Geometry: see drawing. Coordinates: mm, zero at the bounding-box minimum. A direction names the side the tool comes from. Round coordinates to 2 decimals unless told otherwise and drop trailing zeros. Loops run counter-clockwise (first coordinate to the right, second up) from the corner with the lowest first, then second, coordinate; pieces in that order, holes last. Notation, with made-up numbers: (13.25, 15.5) -> (20.25, 15.5) arc R20 ccw to (20.25, 26.5) -> close; hole circle Ø1 at (-5.75, 68). An arc over 180 degrees is marked (long way). Answer in a Markdown table with one row per item.
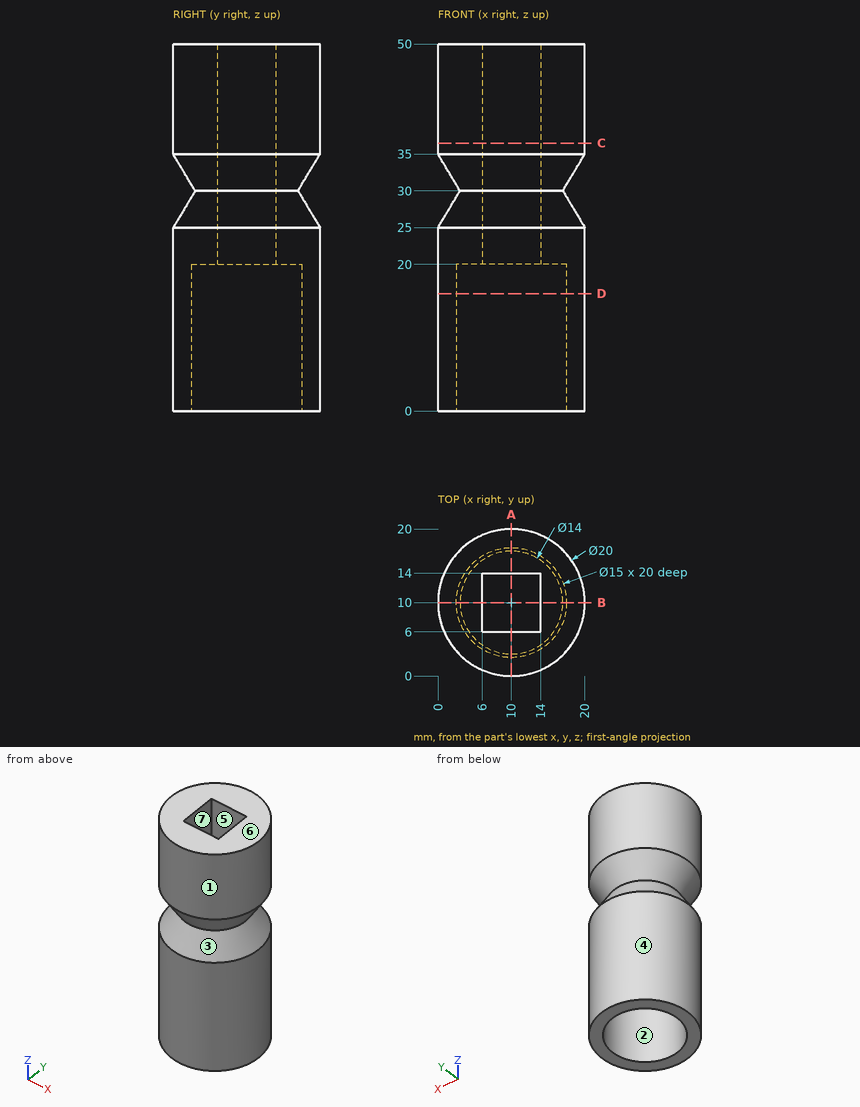
Item 1: Set-up query: the marked faces 1, 2 and 3. Return all of +Z, -Z, +X, -X, +Y, -Y with unobstructed straight access to the full face (end or side cutting, diameter ignored); none if empty.
Ans:
| item | result |
|---|---|
| face 1 | +Z, -Z |
| face 2 | -Z |
| face 3 | none |
Item 2: Section query D-D, the plane z = 16. Output: boundary loops of the cut face in (x, y), and give its area (3 significant figures).
Ans:
| item | result |
|---|---|
| outline | circle Ø20 at (10, 10); hole circle Ø15 at (10, 10) |
| area | 137 mm2 |
Item 3: Ray query, L1, parallel to X at y = 10, z = 10; L2, parallel to Z at x = 5.5, y = 5. Return the intervals inside material, ascending.
Ans:
| item | result |
|---|---|
| L1 | 0 to 2.5, 17.5 to 20 |
| L2 | 20 to 50 |
Item 4: Mould query, pull axis X, two halves, no side actions, for the marked faces 4, 5, 6 and 7. Classes: released by +X, released by -X, zero draft, split by the parting line, or undercut.
Ans:
| item | result |
|---|---|
| face 4 | split by the parting line |
| face 5 | undercut |
| face 6 | zero draft |
| face 7 | undercut |
Item 5: First-contact query: P1, Ø1, axis at y = 17, z = 6.5, coming from the +X side; P2, Ø2.5, axis at y = 8.5, z = 35.5, coming from the -X side; P3, Ø4.5, axis at x = 7.5, y = 8.5, coming from the -Z side. Flat tips, straight axial feed; report the tip coordinate or a pass-through.
Ans:
| item | result |
|---|---|
| P1 | x = 17.6 |
| P2 | x = 0 |
| P3 | z = 20 |
Item 6: Section query C-C, the plane z = 36.5. Output: boundary loops of the cut face in (x, y).
Ans:
| item | result |
|---|---|
| outline | circle Ø20 at (10, 10); hole (6, 6) -> (14, 6) -> (14, 14) -> (6, 14) -> close |
Item 7: Section query A-A, the plane x = 10. Output: boundary loops of the cut face in (y, z).
Ans:
| item | result |
|---|---|
| outline | (0, 0) -> (2.5, 0) -> (2.5, 20) -> (6, 20) -> (6, 50) -> (0, 50) -> (0, 35) -> (3, 30) -> (0, 25) -> close; (14, 20) -> (17.5, 20) -> (17.5, 0) -> (20, 0) -> (20, 25) -> (17, 30) -> (20, 35) -> (20, 50) -> (14, 50) -> close |
